For this review, use the dimensioned drawing (mm, ordinates from the lowest corner) and the shaded views. Round coordinates to 2 decimals unless told otherwise and drop trailing zeros. Loops run counter-clockwise (first coordinate to the right, second up) from the corner with the lowest first, then second, coordinate; pieces in that order, holes last. Notation, with made-up numbers: M 23,-34.75 L 37,-34.75 A7 cw 37,-28.75 Z; hole C 74.25,64 d6. An arc over 180 degrees is marked long. One line per item, written item: value. Start each with the question number.
Item 1: We need section A-A (y = 11.75). Write out the cut boundary in (x, z), then the cut area to 3 significant figures.
Item 2: We need section C-C (z = 3). Write out the cut boundary in (x, y), then the cut area to 3 significant figures.
Item 3: We need section D-D (y = 16.5). Write out the cut boundary in (x, z), then the cut area to 3 significant figures.
Item 4: We need section B-B (x = 3). Write out the cut boundary in (y, z), then the cut area to 3 significant figures.
Item 5: For line 1 along Z through (x, y) = (34, 7); line 2 along X through (y, z) = (5.25, 24); line 3 along Z through (x, y) = (34.5, 4), list the stretches that pass through material, from the lowest coordinate up.
Item 6: Clearance check with flat-ended pins moving along their axes: pin 1 (1.6 mm diameter, centred on x = 34.12, z = 24, fed in from -Y); pin 2 (3 mm diameter, centred on x = 21.5, z = 3.5, fed in from -Y); pin 3 (4.5 mm diameter, centred on x = 3, z = 3, fed in from +Y); pin 4 (3 mm diameter, centred on x = 16.5, z = 14.5, fed in from -Y) (3 decimals). State where each tip first meets the part, or that it passes through.
Item 7: Mouldability with a two-part tool opening along X and no side actions: class the marked faces 1, 2, 3 and 4 as released by +X, released by -X, zero draft, split by the parting line, or undercut.
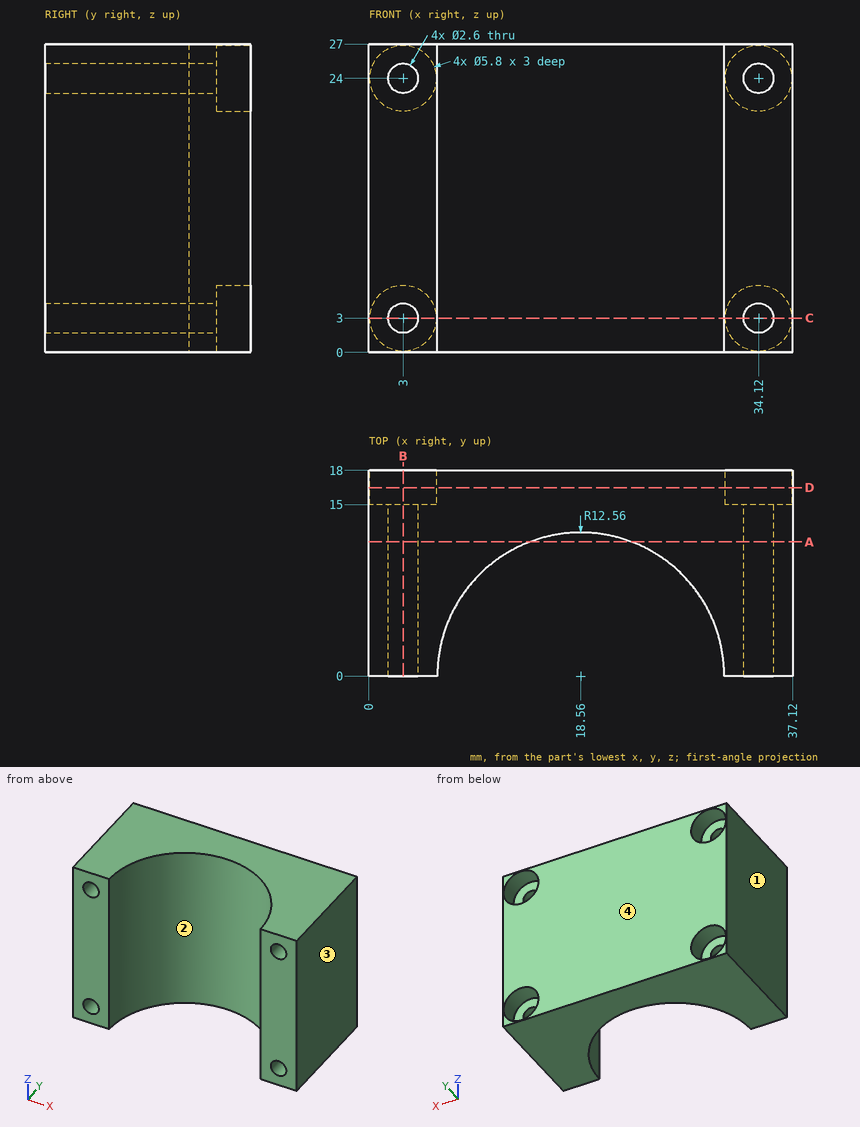
A:
1. outline: M 0,0 L 14.12,0 L 14.12,27 L 0,27 Z; M 23,0 L 37.12,0 L 37.12,27 L 23,27 Z; hole C 3,3 d2.6; hole C 3,24 d2.6; hole C 34.12,3 d2.6; hole C 34.12,24 d2.6
1. area: 741 mm2
2. outline: M 0,0 L 1.7,0 L 1.7,15 L 0.1,15 L 0.1,18 L 0,18 Z; M 4.3,0 L 6,0 A12.56 cw 31.12,0 L 32.82,0 L 32.82,15 L 31.22,15 L 31.22,18 L 5.9,18 L 5.9,15 L 4.3,15 Z; M 35.42,0 L 37.12,0 L 37.12,18 L 37.02,18 L 37.02,15 L 35.42,15 Z
2. area: 308 mm2
3. outline: M 0,0 L 37.12,0 L 37.12,27 L 0,27 Z; hole C 3,3 d5.8; hole C 3,24 d5.8; hole C 34.12,3 d5.8; hole C 34.12,24 d5.8
3. area: 897 mm2
4. outline: M 0,0 L 18,0 L 18,0.1 L 15,0.1 L 15,1.7 L 0,1.7 Z; M 0,4.3 L 15,4.3 L 15,5.9 L 18,5.9 L 18,21.1 L 15,21.1 L 15,22.7 L 0,22.7 Z; M 0,25.3 L 15,25.3 L 15,26.9 L 18,26.9 L 18,27 L 0,27 Z
4. area: 373 mm2
5. line 1: 0 to 1.71, 4.29 to 22.71, 25.29 to 27
5. line 2: 0 to 1.7, 4.3 to 7.15, 29.97 to 32.82, 35.42 to 37.12
5. line 3: 0 to 1.76, 4.24 to 22.76, 25.24 to 27
6. pin 1: through
6. pin 2: y = 11.75
6. pin 3: y = 15
6. pin 4: y = 12.045
7. face 1: released by -X
7. face 2: undercut
7. face 3: released by +X
7. face 4: zero draft
